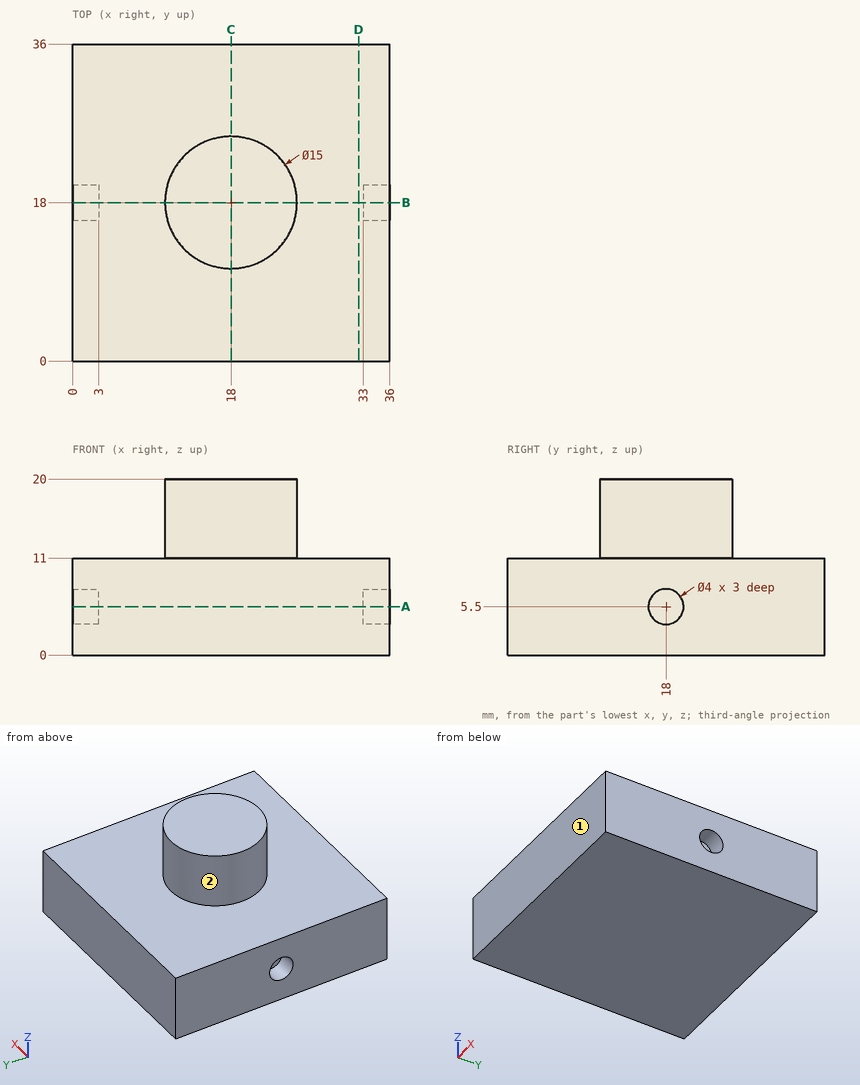
Part print with two shaded views. Sizes in mm from the minimum x, y, z corner. A direction names the side the tool comes from. Give positions to 0.01 mm unless a question says otherwise; leave off trailing zeros. Loops run counter-clockwise (first coordinate to the right, second up) from the corner with the lowest first, then second, coordinate; pieces in that order, holes last. Notation, with made-up numbers: (-31.5, -2.75) - (-7.5, -2.75) arc R28 cw to (-7.5, 19.25) - close; hole circle Ø7 at (-11, 76.25). An arc over 180 degrees is marked (long way). Put each result on its own line as item: value.
Q1. Flat gauge pins, fed straight in: pin 1 (4 mm diameter, centred on y = 22, z = 17.5, fed in from +X); pin 2 (1.2 mm diameter, centred on y = 17, z = 5.5, fed in from +X); pin 3 (2 mm diameter, centred on x = 22, y = 4, fed in from +Z); pin 4 (1 mm diameter, centred on y = 29, z = 12.5, fed in from +X). Where does each tip first touch, or does it go through?
Filled in:
pin 1: stops at x = 25.23
pin 2: stops at x = 33
pin 3: stops at z = 11
pin 4: passes through
Q2. Slice it at C-C (x = 18). Give the cut face in (y, z).
Filled in:
outline: (0, 0) - (36, 0) - (36, 11) - (25.5, 11) - (25.5, 20) - (10.5, 20) - (10.5, 11) - (0, 11) - close
Q3. Slice it at D-D (x = 32.5). Give the cut face in (y, z).
Filled in:
outline: (0, 0) - (36, 0) - (36, 11) - (0, 11) - close
Q4. Tool access for the marked faces 1 and 2: list every direction of +Z, -Z, +X, -X, +Y, -Y with a clear straight run to the whole face (end or side of a thin tool).
Filled in:
face 1: +Z, -Z, +X, -X, -Y
face 2: +Z
Q5. Probe line 1 along Z through (x, y) = (13, 33.5); line 2 along Y through (x, z) = (18, 13); line 3 along X through (y, z) = (14, 18.75). List the from-to ranges inside material, lowest first.
Filled in:
line 1: z = 0 to 11
line 2: y = 10.5 to 25.5
line 3: x = 11.66 to 24.34
Q6. Slice it at A-A (z = 5.5). Give the cut face in (x, y), plus the area to 3 significant figures.
Filled in:
outline: (0, 0) - (36, 0) - (36, 16) - (33, 16) - (33, 20) - (36, 20) - (36, 36) - (0, 36) - (0, 20) - (3, 20) - (3, 16) - (0, 16) - close
area: 1,270 mm²
Q7. Slice it at B-B (y = 18). Give the cut face in (x, z), plus the area to 3 significant figures.
Filled in:
outline: (0, 0) - (36, 0) - (36, 3.5) - (33, 3.5) - (33, 7.5) - (36, 7.5) - (36, 11) - (25.5, 11) - (25.5, 20) - (10.5, 20) - (10.5, 11) - (0, 11) - (0, 7.5) - (3, 7.5) - (3, 3.5) - (0, 3.5) - close
area: 507 mm²
